Read the model definition and answer for the solid it produces. Units are mm, in the model's axes. Face numbers are marked on the shaded views. A direction names the side the tool comes from. Round coordinates to 2 decimals unless told otherwise and drop trailing zeros. Loops run counter-clockwise (first coordinate to the right, second up) from the corner with the lowest first, then second, coordinate; pieces in that order, holes last. Notation, with made-up numbers: (11, 4.25) -> (70, 4.25) arc R12 ccw to (70, 19.25) -> close; hole circle Ø4 at (52, -1.75). An arc over 180 degrees is marked (long way). Put each result on its own line as item: value.
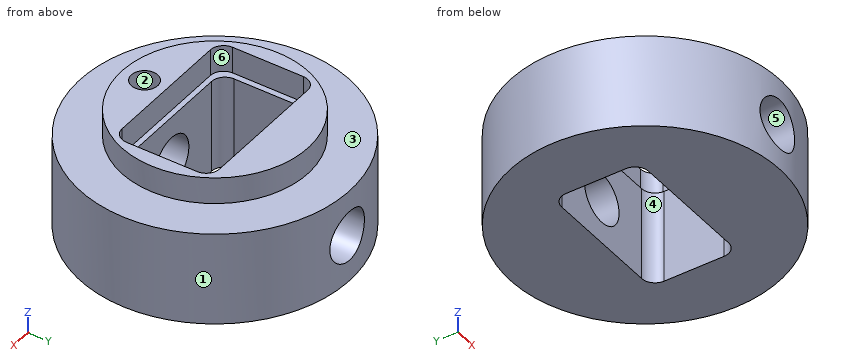
from build123d import *

# Parameters (mm, degrees)
SKETCH_R             = 20.14583
PAD_DEPTH            = 14
SKETCH001_R          = 13.924934
PAD001_DEPTH         = 4
POCKET_DEPTH         = 4
POCKET001_DEPTH      = 18.001
SKETCH004_R          = 3.798047
POCKET002_DEPTH      = 20.14683
POCKET002_DEPTH_BACK = -20.14683
SKETCH005_R          = 1.975009
POCKET003_DEPTH      = 9


with BuildPart() as part:
    # Sketch → Pad (new body)
    with BuildSketch(Plane.XY):
        Circle(SKETCH_R)
    extrude(amount=PAD_DEPTH)

    # Sketch001 (on Face3 of Pad) → Pad001 (join)
    with BuildSketch(Plane.XY.offset(14)):
        Circle(SKETCH001_R)
    extrude(amount=PAD001_DEPTH)

    # Sketch002 (on Face5 of Pad001) → Pocket (cut)
    with BuildSketch(Plane.XY.offset(18)):
        with BuildLine():
            Line((-11.678625, 5.283784), (-11.678625, -5.283784))
            ThreePointArc((-11.678625, -5.283784), (-11.092839, -6.697998), (-9.678625, -7.283784))
            Line((-9.678625, -7.283784), (9.678625, -7.283784))
            ThreePointArc((9.678625, -7.283784), (11.092839, -6.697998), (11.678625, -5.283784))
            Line((11.678625, -5.283784), (11.678625, 5.283784))
            ThreePointArc((11.678625, 5.283784), (11.092839, 6.697998), (9.678625, 7.283784))
            Line((9.678625, 7.283784), (-9.678625, 7.283784))
            ThreePointArc((-9.678625, 7.283784), (-11.092839, 6.697998), (-11.678625, 5.283784))
        make_face()
    extrude(amount=-POCKET_DEPTH, mode=Mode.SUBTRACT)

    # Sketch003 (on Face5 of Pad001) → Pocket001 (cut, through all)
    with BuildSketch(Plane.XY.offset(18)):
        with BuildLine():
            Line((-10.778705, 4.482331), (-10.778705, -4.482331))
            ThreePointArc((-10.778705, -4.482331), (-10.192919, -5.896545), (-8.778705, -6.482331))
            Line((-8.778705, -6.482331), (8.778705, -6.482331))
            ThreePointArc((8.778705, -6.482331), (10.192919, -5.896545), (10.778705, -4.482331))
            Line((10.778705, -4.482331), (10.778705, 4.482331))
            ThreePointArc((10.778705, 4.482331), (10.192919, 5.896545), (8.778705, 6.482331))
            Line((8.778705, 6.482331), (-8.778705, 6.482331))
            ThreePointArc((-8.778705, 6.482331), (-10.192919, 5.896545), (-10.778705, 4.482331))
        make_face()
    extrude(amount=-POCKET001_DEPTH, mode=Mode.SUBTRACT)

    # Sketch004 (on DatumPlane) → Pocket002 (cut, two sides)
    with BuildSketch(Plane(origin=(0, 0, 7), x_dir=(1, 0, 0), z_dir=(0, -1, 0))) as pocket002_sk:
        Circle(SKETCH004_R)
    extrude(amount=-POCKET002_DEPTH, mode=Mode.SUBTRACT)
    extrude(pocket002_sk.sketch, amount=-POCKET002_DEPTH_BACK, mode=Mode.SUBTRACT)

    # Sketch005 (on Face16 of Pocket002) → Pocket003 (cut)
    with BuildSketch(Plane.XY.offset(18)):
        with Locations((0, -10.527462)):
            Circle(SKETCH005_R)
    extrude(amount=-POCKET003_DEPTH, mode=Mode.SUBTRACT)


solid = part.part
Item 1: The part is cut by section C-C (x = 8). Determine the outline of the cut face in (y, z).
Derived:
outline: (-18.49, 0) -> (-6.48, 0) -> (-6.48, 14) -> (-7.28, 14) -> (-7.28, 18) -> (-11.4, 18) -> (-11.4, 14) -> (-18.49, 14) -> close; (6.48, 0) -> (18.49, 0) -> (18.49, 14) -> (11.4, 14) -> (11.4, 18) -> (7.28, 18) -> (7.28, 14) -> (6.48, 14) -> close
Item 2: Which of the six approach directions +Z, -Z, +X, -X, +Y, -Y give full straight-line access (tool end or side, diameter ignored) to the marked faces 4, 5 and 6?
Derived:
face 4: +Z, -Z
face 5: +Y, -Y
face 6: +Z
Item 3: The part is cut by section A-A (x = 0). Determine the outline of the cut face in (y, z).
Derived:
outline: (-20.15, 0) -> (-6.48, 0) -> (-6.48, 3.2) -> (-20.15, 3.2) -> close; (-20.15, 10.8) -> (-12.5, 10.8) -> (-12.5, 18) -> (-13.92, 18) -> (-13.92, 14) -> (-20.15, 14) -> close; (-8.55, 10.8) -> (-6.48, 10.8) -> (-6.48, 14) -> (-7.28, 14) -> (-7.28, 18) -> (-8.55, 18) -> close; (6.48, 0) -> (20.15, 0) -> (20.15, 3.2) -> (6.48, 3.2) -> close; (6.48, 10.8) -> (20.15, 10.8) -> (20.15, 14) -> (13.92, 14) -> (13.92, 18) -> (7.28, 18) -> (7.28, 14) -> (6.48, 14) -> close
Item 4: The part is cut by section B-B (y = -4). Determine the outline of the cut face in (x, z), then the cut area to 3 significant figures.
Derived:
outline: (-19.74, 0) -> (-10.78, 0) -> (-10.78, 14) -> (-11.68, 14) -> (-11.68, 18) -> (-13.34, 18) -> (-13.34, 14) -> (-19.74, 14) -> close; (10.78, 0) -> (19.74, 0) -> (19.74, 14) -> (13.34, 14) -> (13.34, 18) -> (11.68, 18) -> (11.68, 14) -> (10.78, 14) -> close
area: 264 mm^2
Item 5: For a pull along Y with two mould halves and no side action, classify the marked faces 1, 2 and 3 as pulls with the +Y half, pulls with the -Y half, needs draft (parallel to the pull), parting line crosses it, or undercut.
Derived:
face 1: parting line crosses it
face 2: undercut
face 3: needs draft
Item 6: Find the intervals of material crossed by line 1 along Y through (x, z) = (0, 13); line 2 along Z through (x, y) = (0, 11.5); line 3 along Z through (x, y) = (-12, -9.5), in increasing order.
Derived:
line 1: y = -20.15 to -12.5, -8.55 to -6.48, 6.48 to 20.15
line 2: z = 0 to 3.2, 10.8 to 18
line 3: z = 0 to 14
Item 7: The part is cut by section D-D (y = 10). Determine the outline of the cut face in (x, z), then the cut area to 3 significant figures.
Derived:
outline: (-17.49, 0) -> (17.49, 0) -> (17.49, 14) -> (9.69, 14) -> (9.69, 18) -> (-9.69, 18) -> (-9.69, 14) -> (-17.49, 14) -> close; hole circle Ø7.6 at (0, 7)
area: 522 mm^2
Item 8: Flat-ended cylindrical pins translate along their axes: pin 1 Ø3 at (y, z) = (-2.5, 17) entering from +X; pin 2 Ø7 at (x, z) = (0, 7) entering from -Y; pin 3 Ø3 at (x, z) = (-7, 9) entering from -Y; pin 4 Ø3 at (x, z) = (-2, 17) entering from -Y. Find the tip coordinate at first contact, or state that the pin passes through.
Derived:
pin 1: stops at x = 13.89
pin 2: passes through
pin 3: stops at y = -19.38
pin 4: stops at y = -13.92
